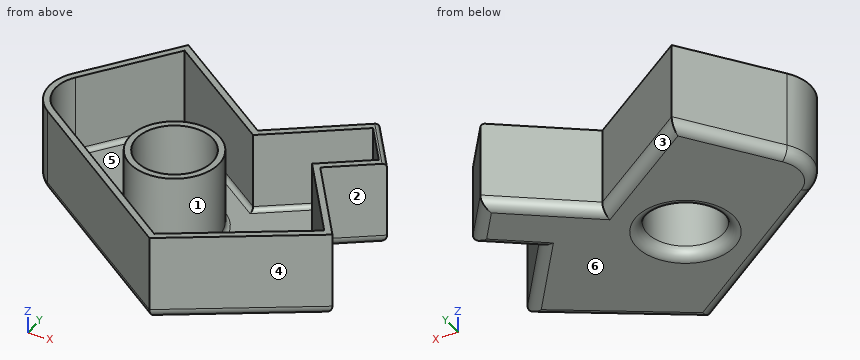
from build123d import *

# Parameters (mm, degrees)
F1_DEPTH      = 40
F2_R          = 17.5
F3_DEPTH      = 71
F3_DEPTH_BACK = 36
F4_T          = -3
F5_R          = 2
F6_R          = 5
F7_R          = 2


with BuildPart() as f1:
    # F0 (on Top) → F1 (new body)
    with BuildSketch(Plane.XY):
        with BuildLine():
            Line((-27.5977612737, 13.564970105), (-82.0387158474, 52.6854230273))
            Line((-82.0387158474, 52.6854230273), (-112.497974617, 11.9829792529))
            ThreePointArc((-112.497974617, 11.9829792529), (-116.2588665454, -3.0005047079), (-108.2223530131, -16.1938193008))
            Line((-108.2223530131, -16.1938193008), (-27.5977612737, -74.6297745564))
            Line((-27.5977612737, -74.6297745564), (35.3226008469, -35.9862801798))
            Line((35.3226008469, -35.9862801798), (7.3407227042, 3.188352482))
            Line((7.3407227042, 3.188352482), (29.3764571995, 18.9281615252))
            Line((29.3764571995, 18.9281615252), (12.6650570628, 42.3241236648))
            Line((12.6650570628, 42.3241236648), (-27.5977612737, 13.564970105))
        make_face()
    extrude(amount=-F1_DEPTH)

    # F2 (on Top) → F3 (cut, two sides)
    with BuildSketch(Plane.XY) as f3_sk:
        with Locations((-49.8492009938, -15.0985578075)):
            Circle(F2_R)
    extrude(amount=-F3_DEPTH, mode=Mode.SUBTRACT)
    extrude(f3_sk.sketch, amount=F3_DEPTH_BACK, mode=Mode.SUBTRACT)

    # F4
    f4_openings = [f1.faces().sort_by_distance(p)[0] for p in [
        (-66.747329, -43.807571, 0),
    ]]
    offset(amount=F4_T, openings=f4_openings, kind=Kind.INTERSECTION)

    # F5
    f5_edges = [f1.edges().sort_by_distance(p)[0] for p in [
        (-95.747934, 29.358811, -37),
        (-113.29282, -2.550429, -37),
        (-66.960878, -42.394636, -37),
        (1.776075, -53.068764, -37),
        (17.083964, -15.613582, -37),
        (14.173675, 11.755743, -37),
        (18.579557, 28.882428, -37),
        (-7.817716, 24.006862, -37),
        (-54.501405, 29.203302, -37),
        (-70.349201, -15.098558, -37),
    ]]
    fillet(f5_edges, radius=F5_R)

    # F6
    f6_edges = [f1.edges().sort_by_distance(p)[0] for p in [
        (-67.910057, -45.411797, -40),
        (-116.258867, -3.000505, -40),
        (3.86242, -55.308027, -40),
        (-97.268345, 32.334201, -40),
        (21.331662, -16.398964, -40),
        (-54.818239, 33.125197, -40),
        (18.35859, 11.058257, -40),
        (-7.466352, 27.944547, -40),
        (21.020757, 30.626143, -40),
        (-67.349201, -15.098558, -40),
    ]]
    fillet(f6_edges, radius=F6_R)

    # F7
    f7_edges = [f1.edges().sort_by_distance(p)[0] for p in [
        (21.020757, 30.626143, 0),
    ]]
    fillet(f7_edges, radius=F7_R)


solid = f1.part
Verification items for the finished model (mm, model axes). Face numbers are marked on the shaded views. A direction names the side the tool comes from. Coordinates: 2 decimals unless noted, no trailing zeros. Write each loop counter-clockwise with the first axis right and the second up, starting at its lowest first coordinate (ties: lowest second). Pieces come first, ordered by that corner, then holes. Notation, with made-up numbers: M 3,41 L 37,41 A27 ccw 37,78 Z; hole C 83,-13 d8. An arc over 180 degrees is marked long. One line per question, with ' | ' between items.
1) Material ranges on L1, parallel to Y at x = -66, z = -33; L2, parallel to X at y = 15, z = -25.5; L3, parallel to X at y = 42, z = -20, recorded low to high.
Solutions:
L1: -46.8 to -43.09, -27.72 to -21.84, -8.36 to -2.47, 37.47 to 41.16 | L2: -110.24 to -106.49, -34.74 to -29.59, -25.59 to -20.43, 18.72 to 23.88 | L3: -90.04 to -86.29, -72.31 to -67.17, 12.21 to 12.9
2) Sectioned sample at A-A on z = -23.5. Record the cut outline in (x, y), then the cut area to 3 significant figures.
Solutions:
outline: M -112.5,11.98 A20 ccw -108.22,-16.19 L -27.6,-74.63 L 35.32,-35.99 L 7.34,3.19 L 29.38,18.93 L 12.67,42.32 L -27.6,13.56 L -82.04,52.69 Z; C -49.85,-15.1 d41; hole M -110.1,10.19 A17 ccw -106.46,-13.76 L -27.46,-71.02 L 31.01,-35.11 L 3.16,3.89 L 25.19,19.63 L 11.97,38.14 L -27.6,9.87 L -81.4,48.53 Z; hole C -49.85,-15.1 d35 | area: 1,750 mm^2
3) Depth check by flat-ended pin: pin 1 Ø5 at (y, z) = (3, -4.5) entering from +X; pin 2 Ø3 at (x, z) = (-86.5, -18) entering from +Y; pin 3 Ø5 at (x, z) = (11, -30.5) entering from -Y; pin 4 Ø5 at (x, y) = (-89, 39.5) entering from +Z. Enter the tip coordinate at first touch or a pass-through.
Solutions:
pin 1: x = 10.58 | pin 2: y = 48.73 | pin 3: y = -52.46 | pin 4: z = 0
4) Access from +Z, -Z, +X, -X, +Y, -Y to the whole of each face (thin tool, end or side, straight path). Record for the marked faces 1, 2 and 3.
Solutions:
face 1: +Z | face 2: +Z, -Z, +X | face 3: -Z, +Y
5) Release check for a two-part mould opening along X. For the marked faces 4, 5 and 6 record: +X half, -X half, draft (parallel to the pull), parting line (faces both ways), or undercut.
Solutions:
face 4: +X half | face 5: undercut | face 6: draft
